Read the model definition and answer for the solid it produces. Units are mm, in the model's axes. A direction names the side the tool comes from. Give positions to 0.01 mm unless a question says otherwise; leave off trailing zeros. Write each loop counter-clockwise with the first axis right and the second up, starting at its lowest first coordinate (ties: lowest second). Pieces come first, ordered by that corner, then holes. Notation, with made-up numbers: (59.25, -20) - (83.25, -20) arc R23 ccw to (83.25, 16) - close; hole circle Ø1 at (-40, 9.5). An arc over 180 degrees is marked (long way). Answer as CSV lines item,"result".
Autodesk Inventor part; units mm, degrees
ref_plane "Work Plane1" through (0, 0, 28.55) normal (0, 0, -1) x (-1, 0, 0)
ref_plane "YZ Plane" through (0, 0, 0) normal (1, 0, 0) x (0, 1, 0)
ref_plane "XZ Plane" through (0, 0, 0) normal (0, 1, 0) x (-1, 0, 0)
sketch "Sketch1" plane through (0, 0, 0) normal (0, 0, 1) x (1, 0, 0)
  circle A0 centre (0, 0) radius 4
  dimension "d0" = 8
extrude "Extrusion1" add sketch "Sketch1" along normal blind 235
sketch "Sketch5" plane through (0, 0, 235) normal (0, 0, 1) x (1, 0, 0)
  circle A0 centre (0, 0) radius 4
  line L0 (-3.4641, 2) -> (3.4641, 2)
  arc A1 (3.4641, 2) -> (-3.4641, 2) centre (0, 0) ccw
  dimension "d18" = 2
extrude "Extrusion5" cut sketch "Sketch5" against normal blind 40 contours L0 A0 picked at (-0.1548, 2.6577)
sketch "Sketch7" plane through (-3.4641, 2, 235) normal (0, 1, 0) x (1, 0, 0)
  circle A0 centre (3.4641, 209.45) radius 1.5
  circle A1 centre (3.4641, 212.2) radius 1.5
  line L0 (1.9641, 209.45) -> (1.9641, 212.2)
  line L1 (4.9641, 209.45) -> (4.9641, 212.2)
  line L2 (-0.5359, 235) -> (-0.5359, 0)
  line L3 (7.4641, 235) -> (7.4641, 0)
  line L4 (-0.5359, 191) -> (7.4641, 191)
  line L5 (7.4641, 191) -> (7.4641, 171)
  line L6 (7.4641, 171) -> (-0.5359, 171)
  line L7 (-0.5359, 171) -> (-0.5359, 191)
  point P0 (3.4641, 235)
  dimension "d21" = 3
  dimension "d22" = 3
  dimension "d23" = 2.75
  dimension "d24" = 22.8
  dimension "d25" = 20
  dimension "d26" = 44
extrude "Extrusion6" cut sketch "Sketch7" along normal through all
ref_plane "Work Plane1" through (0, 0, 28.55) normal (0, 0, -1) x (-1, 0, 0)
sketch "Sketch8" plane through (0, 0, 28.55) normal (0, 0, -1) x (-1, 0, 0)
  circle A0 centre (0, 0) radius 4
  circle A1 centre (0, 0) radius 3.2
  dimension "d30" = 0.8
extrude "Extrusion7" cut sketch "Sketch8" against normal blind 1
properties part number "AA054" material "Aluminum 6061"
(1) A cutting plane is placed at A-A (x = 0). Write down the section's boundary in (y, z).
Worked out:
outline,"(-4, 0) - (4, 0) - (4, 21.3) - (2, 21.3) - (2, 27.05) - (4, 27.05) - (4, 28.55) - (3.2, 28.55) - (3.2, 29.55) - (4, 29.55) - (4, 44) - (2, 44) - (2, 64) - (4, 64) - (4, 195) - (2, 195) - (2, 235) - (-4, 235) - (-4, 29.55) - (-3.2, 29.55) - (-3.2, 28.55) - (-4, 28.55) - close"
(2) Each of these flat-tipped pins is pushed along its axis until it touches: P1, Ø2.5, axis at x = 0, z = 24.5, coming from the +Y side; P2, Ø1, axis at x = -1.5, y = 3.5, coming from the +Z side; P3, Ø1.4, axis at y = 3, z = 24.5, coming from the -X side. Where does it stop, or does it pass through?
Worked out:
P1,"stops at y = 2"
P2,"stops at z = 195"
P3,"stops at x = -3.27"
(3) Find the intervals of material crossed by L1, parallel to Z at x = -2.25, y = 3; L2, parallel to Z at x = -0.5, y = 2.75; L3, parallel to X at y = -0.5, z = 209, in increasing order.
Worked out:
L1,"z = 0 to 28.55, 29.55 to 44, 64 to 195"
L2,"z = 0 to 21.39, 26.96 to 44, 64 to 195"
L3,"x = -3.97 to 3.97"
(4) The mould has two halves that part along Z. Classify faces 5 (the cylindrical face through (2.539, -1.947, 29.043)), 6 (the cylindrical face through (2.15, -3.373, 130.837)), 7 (the flat face through (0, 0, 235)): +Z half, -Z half, draft (parallel to the pull), parting line (faces both ways), or undercut.
Worked out:
face 5,"undercut"
face 6,"draft"
face 7,"+Z half"
(5) A cutting plane is placed at B-B (z = 41.5). Write down the section's boundary in (x, y).
Worked out:
outline,"circle Ø8 at (0, 0)"
(6) For faces 1 (the flat face through (0, 2, 215)), 2 (the cylindrical face through (2.15, -3.373, 14.075)), 3 (the flat face through (2, 3, 28.55)), 4 (the flat face through (0, 2, 54)), determine the directions among +Z, -Z, +X, -X, +Y, -Y from which every point of the face is accessible in a straight line to the end or side of a thin tool.
Worked out:
face 1,"+Z, +X, -X, +Y"
face 2,"+Z, -Z"
face 3,"none"
face 4,"+X, -X, +Y"
